Geometry check sheet. Reference: the model listing, model coordinates, mm. Coordinates: 2 decimals unless noted, no trailing zeros. Write each loop counter-clockwise with the first axis right and the second up, starting at its lowest first coordinate (ties: lowest second). Pieces come first, ordered by that corner, then holes. Notation, with made-up numbers: (-13.75, 64.25) -> (17.25, 64.25) arc R25 cw to (17.25, 80.25) -> close; hole circle Ø8 at (-7, 56.25). An arc over 180 degrees is marked (long way). Answer as CSV lines item,"result".
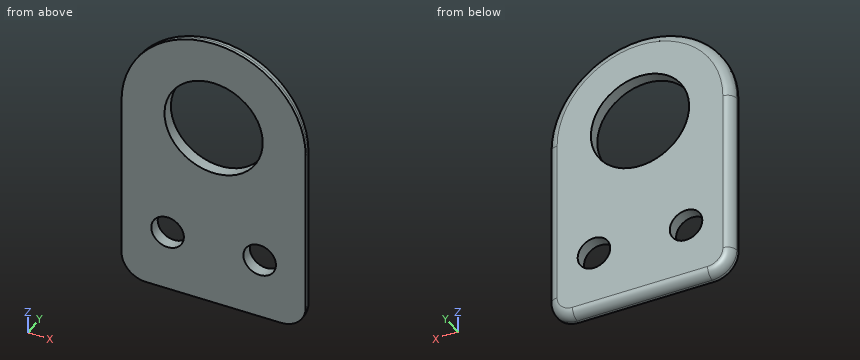
```python
from build123d import *

# Parameters (mm, degrees)
SKETCH1_R            = 8
BOSS_EXTRUDE1_DEPTH  = 2
M5_CLEARANCE_HOLE1_D = 5.3
FILLET1_R            = 4
FILLET2_R            = 1.5


with BuildPart() as part:
    # Sketch1 → Boss-Extrude1 (new body)
    with BuildSketch(Plane(origin=(0, 0, 0), x_dir=(1, 0, 0), z_dir=(0, 1, 0))):
        with BuildLine():
            Line((-15, 0), (-15, 31))
            Line((-15, 31), (15, 31))
            Line((15, 31), (15, 0))
            ThreePointArc((15, 0), (0, -15), (-15, 0))
        make_face()
        with Locations(Location((0, 0, 0), (0, 0, 270))):
            Circle(SKETCH1_R, mode=Mode.SUBTRACT)
    extrude(amount=BOSS_EXTRUDE1_DEPTH)

    # M5 Clearance Hole1 (through all)
    with Locations(Plane(origin=(-7.5, 2, -21), x_dir=(0, 0, 1), z_dir=(0, 1, 0))):
        with Locations((0, 0), (0, 15)):
            Hole(M5_CLEARANCE_HOLE1_D / 2)

    # Fillet1
    fillet1_edges = [part.edges().sort_by_distance(p)[0] for p in [
        (-15, 1, -31),
        (15, 1, -31),
    ]]
    fillet(fillet1_edges, radius=FILLET1_R)

    # Fillet2
    fillet2_edges = [part.edges().sort_by_distance(p)[0] for p in [
        (15, 2, -13.5),
        (-15, 2, -13.5),
        (0, 2, -31),
        (-13.828427125, 2, -29.828427125),
        (13.828427125, 2, -29.828427125),
        (0, 2, 15),
    ]]
    fillet(fillet2_edges, radius=FILLET2_R)


solid = part.part
```
Item 1: Cross-section at B-B, the plane z = -21. Record the cut outline in (x, y).
Responses:
outline,"(-15, 0) -> (-10.15, 0) -> (-10.15, 2) -> (-13.5, 2) arc R1.5 ccw to (-15, 0.5) -> close; (-4.85, 0) -> (4.85, 0) -> (4.85, 2) -> (-4.85, 2) -> close; (10.15, 0) -> (15, 0) -> (15, 0.5) arc R1.5 ccw to (13.5, 2) -> (10.15, 2) -> close"
Item 2: Cross-section at A-A, the plane y = 1.7. Record the cut outline in (x, z).
Responses:
outline,"(-14.4, -27) arc R3.4 ccw to (-11, -30.4) -> (11, -30.4) arc R3.4 ccw to (14.4, -27) -> (14.4, 0) arc R14.4 ccw to (-14.4, 0) -> close; hole circle Ø5.3 at (-7.5, -21); hole circle Ø16 at (0, 0); hole circle Ø5.3 at (7.5, -21)"
Item 3: Thickness scan on probe 1 along X at (y, z) = (1.4, -21); probe 2 along Z at (x, y) = (7, 1); probe 3 along Z at (x, y) = (5.25, 0.2). Record the ranges inside material, lowest first.
Responses:
probe 1,"x = -14.7 to -10.15, -4.85 to 4.85, 10.15 to 14.7"
probe 2,"z = -30.91 to -23.6, -18.4 to -3.87, 3.87 to 13.17"
probe 3,"z = -31 to -22.4, -19.6 to -6.04, 6.04 to 14.05"
Item 4: Cross-section at C-C, the plane z = -0.5. Record the cut outline in (x, y), plus the area to 3 significant figures.
Responses:
outline,"(-15, 0) -> (-7.98, 0) -> (-7.98, 2) -> (-13.5, 2) arc R1.5 ccw to (-15, 0.5) -> close; (7.98, 0) -> (15, 0) -> (15, 0.5) arc R1.5 ccw to (13.5, 2) -> (7.98, 2) -> close"
area,"27.1 mm2"
Item 5: Cross-section at D-D, the plane x = -7.5. Count the separate pieces of the cut face and the enclosed holes in it, plus the area to 3 significant figures.
Responses:
separate pieces,"3"
enclosed holes,"0"
area,"65.2 mm2"
